```python
from build123d import *

# Parameters (mm, degrees)
SKETCH_1_W           = 100
SKETCH_1_H           = 80
EXTRUDE_1_DEPTH      = 39
SKETCH_2_W           = 3.287907932
SKETCH_2_H           = 80
CUT_EXTRUDE_1_DEPTH  = 15
SKETCH_3_W           = 13.487907932
SKETCH_3_H           = 8
CUT_EXTRUDE_2_DEPTH  = 21
SKETCH_3_2_W         = 13.487907932
SKETCH_3_2_H         = 8
CUT_EXTRUDE_3_DEPTH  = 15
SKETCH_4_W           = 13.487907932
SKETCH_4_H           = 8
CUT_EXTRUDE_4_DEPTH  = 21
SKETCH_4_3_W         = 13.487907932
SKETCH_4_3_H         = 8
CUT_EXTRUDE_5_DEPTH  = 15
SKETCH_5_W           = 13.487907932
SKETCH_5_H           = 8
CUT_EXTRUDE_6_DEPTH  = 21
SKETCH_5_2_W         = 13.487907932
SKETCH_5_2_H         = 8
CUT_EXTRUDE_7_DEPTH  = 15
SKETCH_6_W           = 13.487907932
SKETCH_6_H           = 8
CUT_EXTRUDE_8_DEPTH  = 21
SKETCH_6_2_W         = 13.487907932
SKETCH_6_2_H         = 8
CUT_EXTRUDE_9_DEPTH  = 36
SKETCH_7_R           = 2.05
CUT_EXTRUDE_10_DEPTH = 3
SKETCH_8_R           = 2.05
CUT_EXTRUDE_11_DEPTH = 3
SKETCH_9_R           = 2.05
CUT_EXTRUDE_12_DEPTH = 3
SKETCH_10_R          = 2.05
CUT_EXTRUDE_13_DEPTH = 3
SKETCH_11_W          = 40
SKETCH_11_H          = 20
CUT_EXTRUDE_14_DEPTH = 10
SKETCH_12_R          = 2.5
EXTRUDE_2_DEPTH      = 10


with BuildPart() as part:
    # Sketch 1 → Extrude 1 (new body)
    with BuildSketch(Plane(origin=(0, 0, 0), x_dir=(1, 0, 0), z_dir=(0, 1, 0))):
        Rectangle(SKETCH_1_W, SKETCH_1_H)
    extrude(amount=EXTRUDE_1_DEPTH)

    # Sketch 2 → Cut-Extrude 1 (cut)
    with BuildSketch(Plane(origin=(0, 39, 0), x_dir=(1, 0, 0), z_dir=(0, 1, 0))):
        with Locations((-48.356046034, 0)):
            Rectangle(SKETCH_2_W, SKETCH_2_H)
        with Locations((-43.256046034, 0)):
            Rectangle(SKETCH_2_W, SKETCH_2_H)
        with Locations((-38.156046034, 0)):
            Rectangle(SKETCH_2_W, SKETCH_2_H)
        with Locations((-33.056046034, 0)):
            Rectangle(SKETCH_2_W, SKETCH_2_H)
        with Locations((-27.956046034, 0)):
            Rectangle(SKETCH_2_W, SKETCH_2_H)
        with Locations((-22.856046034, 0)):
            Rectangle(SKETCH_2_W, SKETCH_2_H)
        with Locations((-17.756046034, 0)):
            Rectangle(SKETCH_2_W, SKETCH_2_H)
        with Locations((-12.656046034, 0)):
            Rectangle(SKETCH_2_W, SKETCH_2_H)
        with Locations((-7.556046034, 0)):
            Rectangle(SKETCH_2_W, SKETCH_2_H)
        with Locations((-2.456046034, 0)):
            Rectangle(SKETCH_2_W, SKETCH_2_H)
        with Locations((2.643953966, 0)):
            Rectangle(SKETCH_2_W, SKETCH_2_H)
        with Locations((7.743953966, 0)):
            Rectangle(SKETCH_2_W, SKETCH_2_H)
        with Locations((12.843953966, 0)):
            Rectangle(SKETCH_2_W, SKETCH_2_H)
        with Locations((17.943953966, 0)):
            Rectangle(SKETCH_2_W, SKETCH_2_H)
        with Locations((23.043953966, 0)):
            Rectangle(SKETCH_2_W, SKETCH_2_H)
        with Locations((28.143953966, 0)):
            Rectangle(SKETCH_2_W, SKETCH_2_H)
        with Locations((33.243953966, 0)):
            Rectangle(SKETCH_2_W, SKETCH_2_H)
        with Locations((38.343953966, 0)):
            Rectangle(SKETCH_2_W, SKETCH_2_H)
        with Locations((43.443953966, 0)):
            Rectangle(SKETCH_2_W, SKETCH_2_H)
        with Locations((48.543953966, 0)):
            Rectangle(SKETCH_2_W, SKETCH_2_H)
    extrude(amount=-CUT_EXTRUDE_1_DEPTH, mode=Mode.SUBTRACT)

    # Sketch 3 → Cut-Extrude 2 (cut)
    with BuildSketch(Plane(origin=(0, 24, 0), x_dir=(1, 0, 0), z_dir=(0, 1, 0))):
        with Locations((-33.056046034, 36)):
            Rectangle(SKETCH_3_W, SKETCH_3_H)
    extrude(amount=-CUT_EXTRUDE_2_DEPTH, mode=Mode.SUBTRACT)

    # Sketch 3_2 → Cut-Extrude 3 (cut)
    with BuildSketch(Plane(origin=(0, 24, 0), x_dir=(1, 0, 0), z_dir=(0, 1, 0))):
        with Locations((-33.056046034, 36)):
            Rectangle(SKETCH_3_2_W, SKETCH_3_2_H)
    extrude(amount=CUT_EXTRUDE_3_DEPTH, mode=Mode.SUBTRACT)

    # Sketch 4 → Cut-Extrude 4 (cut)
    with BuildSketch(Plane(origin=(0, 24, 0), x_dir=(1, 0, 0), z_dir=(0, 1, 0))):
        with Locations((33.243953966, 36)):
            Rectangle(SKETCH_4_W, SKETCH_4_H)
    extrude(amount=-CUT_EXTRUDE_4_DEPTH, mode=Mode.SUBTRACT)

    # Sketch 4_3 → Cut-Extrude 5 (cut)
    with BuildSketch(Plane(origin=(0, 24, 0), x_dir=(1, 0, 0), z_dir=(0, 1, 0))):
        with Locations((33.243953966, 36)):
            Rectangle(SKETCH_4_3_W, SKETCH_4_3_H)
    extrude(amount=CUT_EXTRUDE_5_DEPTH, mode=Mode.SUBTRACT)

    # Sketch 5 → Cut-Extrude 6 (cut)
    with BuildSketch(Plane(origin=(0, 24, 0), x_dir=(1, 0, 0), z_dir=(0, 1, 0))):
        with Locations((-33.056046034, -36)):
            Rectangle(SKETCH_5_W, SKETCH_5_H)
    extrude(amount=-CUT_EXTRUDE_6_DEPTH, mode=Mode.SUBTRACT)

    # Sketch 5_2 → Cut-Extrude 7 (cut)
    with BuildSketch(Plane(origin=(0, 24, 0), x_dir=(1, 0, 0), z_dir=(0, 1, 0))):
        with Locations((-33.056046034, -36)):
            Rectangle(SKETCH_5_2_W, SKETCH_5_2_H)
    extrude(amount=CUT_EXTRUDE_7_DEPTH, mode=Mode.SUBTRACT)

    # Sketch 6 → Cut-Extrude 8 (cut)
    with BuildSketch(Plane(origin=(0, 39, 0), x_dir=(1, 0, 0), z_dir=(0, 1, 0))):
        with Locations((33.243953966, -36)):
            Rectangle(SKETCH_6_W, SKETCH_6_H)
    extrude(amount=-CUT_EXTRUDE_8_DEPTH, mode=Mode.SUBTRACT)

    # Sketch 6_2 → Cut-Extrude 9 (cut)
    with BuildSketch(Plane(origin=(0, 39, 0), x_dir=(1, 0, 0), z_dir=(0, 1, 0))):
        with Locations((33.243953966, -36)):
            Rectangle(SKETCH_6_2_W, SKETCH_6_2_H)
    extrude(amount=-CUT_EXTRUDE_9_DEPTH, mode=Mode.SUBTRACT)

    # Sketch 7 → Cut-Extrude 10 (cut)
    with BuildSketch(Plane(origin=(0, 3, 0), x_dir=(1, 0, 0), z_dir=(0, 1, 0))):
        with Locations(Location((-33.395851618, 36.021594171, 0), (0, 0, 270))):
            Circle(SKETCH_7_R)
    extrude(amount=-CUT_EXTRUDE_10_DEPTH, mode=Mode.SUBTRACT)

    # Sketch 8 → Cut-Extrude 11 (cut)
    with BuildSketch(Plane(origin=(0, 3, 0), x_dir=(1, 0, 0), z_dir=(0, 1, 0))):
        with Locations(Location((33.312820736, 35.94065507, 0), (0, 0, 270))):
            Circle(SKETCH_8_R)
    extrude(amount=-CUT_EXTRUDE_11_DEPTH, mode=Mode.SUBTRACT)

    # Sketch 9 → Cut-Extrude 12 (cut)
    with BuildSketch(Plane(origin=(0, 3, 0), x_dir=(1, 0, 0), z_dir=(0, 1, 0))):
        with Locations(Location((-32.970812698, -36.238015002, 0), (0, 0, 270))):
            Circle(SKETCH_9_R)
    extrude(amount=-CUT_EXTRUDE_12_DEPTH, mode=Mode.SUBTRACT)

    # Sketch 10 → Cut-Extrude 13 (cut)
    with BuildSketch(Plane(origin=(0, 3, 0), x_dir=(1, 0, 0), z_dir=(0, 1, 0))):
        with Locations(Location((33.252132878, -36.225040763, 0), (0, 0, 270))):
            Circle(SKETCH_10_R)
    extrude(amount=-CUT_EXTRUDE_13_DEPTH, mode=Mode.SUBTRACT)

    # Sketch 11 → Cut-Extrude 14 (cut)
    with BuildSketch(Plane(origin=(50, 0, 0), x_dir=(0, 0, -1), z_dir=(1, 0, 0))):
        Rectangle(SKETCH_11_W, SKETCH_11_H)
    extrude(amount=-CUT_EXTRUDE_14_DEPTH, mode=Mode.SUBTRACT)

    # Sketch 12 → Extrude 2 (add)
    with BuildSketch(Plane(origin=(40, 0, 0), x_dir=(0, 0, -1), z_dir=(1, 0, 0))):
        with Locations((-15.422086217, 4.286980586)):
            Circle(SKETCH_12_R)
        with Locations((-6.396528349, 4.286980586)):
            Circle(SKETCH_12_R)
        with Locations((4.962166927, 4.286980586)):
            Circle(SKETCH_12_R)
        with Locations((14.417513265, 4.286980586)):
            Circle(SKETCH_12_R)
    extrude(amount=EXTRUDE_2_DEPTH)


solid = part.part
```
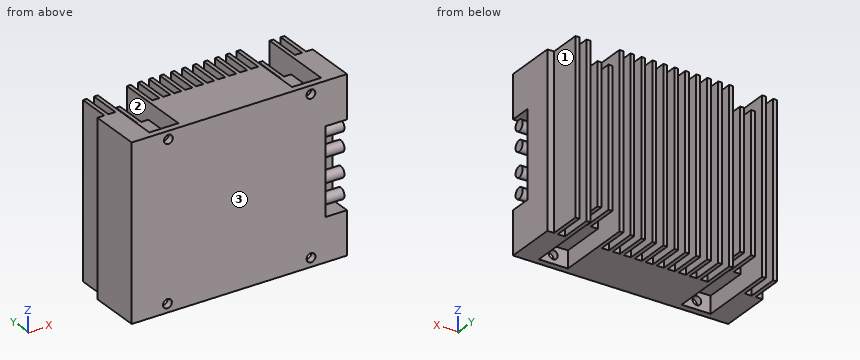
Read the model definition and answer for the solid it produces. Units are mm, in the model's axes. Face numbers are marked on the shaded views. Give positions to 0.01 mm unless a question says otherwise; leave off trailing zeros. Write each loop counter-clockwise with the first axis right and the second up, starting at its lowest first coordinate (ties: lowest second). Pieces come first, ordered by that corner, then holes. Notation, with made-up numbers: (61.5, -33.75) -> (104.5, -33.75) arc R20 ccw to (104.5, -2.75) -> close; hole circle Ø9 at (84, 19). An arc over 180 degrees is marked (long way). Answer as a JSON object with one key per item and string values.
1) Section B-B on x = 38.5 is taken. Write down the section's boundary in (y, z), then the cut area to 3 significant figures.
Findings below:
{"outline": "(0, -40) -> (3, -40) -> (3, -32) -> (24, -32) -> (24, 32) -> (3, 32) -> (3, 40) -> (0, 40) -> close", "area": "1,580 mm^2"}
2) For a pull along X with two mould halves and no side action, classify the marked faces 1, 2 and 3 as pulls with the +X half, pulls with the -X half, needs draft (parallel to the pull), parting line crosses it, or undercut.
Findings below:
{"face 1": "pulls with the +X half", "face 2": "undercut", "face 3": "needs draft"}
3) Flat-ended cylindrical pins translate along their axes: pin 1 Ø2 at (x, y) = (34, 34.5) entering from +Z; pin 2 Ø2.5 at (x, z) = (33, 7) entering from +Y; pin 3 Ø4 at (x, y) = (32.5, 20) entering from -Z; pin 4 Ø2.5 at (x, z) = (33.25, 36.23) entering from +Y. Find the tip coordinate at first contact, or state that the pin passes through.
Findings below:
{"pin 1": "stops at z = 32", "pin 2": "stops at y = 24", "pin 3": "stops at z = -32", "pin 4": "passes through"}
4) Section D-D on y = 22.5 is taken. Write down the section's boundary in (x, z).
Findings below:
{"outline": "(-50, -40) -> (-39.8, -40) -> (-39.8, -32) -> (-26.31, -32) -> (-26.31, -40) -> (26.5, -40) -> (26.5, -32) -> (39.99, -32) -> (39.99, -40) -> (50, -40) -> (50, 40) -> (39.99, 40) -> (39.99, 32) -> (26.5, 32) -> (26.5, 40) -> (-26.31, 40) -> (-26.31, 32) -> (-39.8, 32) -> (-39.8, 40) -> (-50, 40) -> close"}
5) Section C-C on y = 31 is taken. Count the separate pieces of the cut face and the enclosed holes in it, then the cut area to 3 significant figures.
Findings below:
{"separate pieces": "19", "enclosed holes": "0", "area": "2,640 mm^2"}
6) Straight lines are drawn through the part: probe 1 along X at (y, z) = (4, -36); probe 2 along Z at (x, y) = (44.5, 3.5); probe 3 along Y at (x, z) = (43, -29.5). For each, find the intervals that lie inside material, in ascending order. Write a range as from..to.
Findings below:
{"probe 1": "x = -50..-39.8, -26.31..26.5, 39.99..50", "probe 2": "z = -40..-20, -16.79..-12.04, -7.34..-2.59, 4.02..8.77, 13.05..17.79, 20..40", "probe 3": "y = 0..24"}
7) Section A-A on y = 8.5 is taken. Write down the section's boundary in (x, z), then the cut area to 3 significant figures.
Findings below:
{"outline": "(-50, -40) -> (-39.8, -40) -> (-39.8, -32) -> (-26.31, -32) -> (-26.31, -40) -> (26.5, -40) -> (26.5, -32) -> (39.99, -32) -> (39.99, -40) -> (50, -40) -> (50, -20) -> (40, -20) -> (40, 20) -> (50, 20) -> (50, 40) -> (39.99, 40) -> (39.99, 32) -> (26.5, 32) -> (26.5, 40) -> (-26.31, 40) -> (-26.31, 32) -> (-39.8, 32) -> (-39.8, 40) -> (-50, 40) -> close", "area": "7,170 mm^2"}
